```python
from build123d import *

# Parameters (mm, degrees)
SKETCH001_W                   = 50
SKETCH001_H                   = 60
PAD001_DEPTH                  = 17.5
THICKNESS_T                   = -2.5
SKETCH002_R                   = 2.5
PAD002_DEPTH                  = 17.45
SKETCH003_R                   = 0.4
POCKET_DEPTH                  = 1
SKETCH004_W                   = 7
SKETCH004_H                   = 7
PAD003_DEPTH                  = 15
SKETCH004_MIRRORED_2_W        = 7
SKETCH004_MIRRORED_2_H        = 7
PAD003_MIRRORED_2_DEPTH       = 15
SKETCH005_R                   = 1.25
POCKET001_DEPTH               = 12.5
SKETCH005_MIRRORED002_2_R     = 1.25
POCKET001_MIRRORED002_2_DEPTH = 12.5
POCKET002_DEPTH               = 2.5
SKETCH007_W                   = 9
SKETCH007_H                   = 7
POCKET003_DEPTH               = 2.5
FILLET_R                      = 3
FILLET001_R                   = 2
FILLET002_R                   = 1
FILLET003_R                   = 1
FILLET004_R                   = 1
FILLET005_R                   = 1


with BuildPart() as part:
    # Sketch001 → Pad001 (new body)
    with BuildSketch(Plane.XY):
        Rectangle(SKETCH001_W, SKETCH001_H)
    extrude(amount=PAD001_DEPTH)

    # Thickness
    thickness_openings = [part.faces().sort_by_distance(p)[0] for p in [
        (0, 0, 17.5),
    ]]
    offset(amount=THICKNESS_T, openings=thickness_openings)

    # Sketch002 (on Face11 of Thickness) → Pad002 (join)
    with BuildSketch(Plane.XY.offset(2.5)):
        with Locations((-10.415, -7.665)):
            Circle(SKETCH002_R)
        with Locations((-1.695, 13.555)):
            Circle(SKETCH002_R)
    extrude(amount=PAD002_DEPTH)

    # Sketch003 (on Face14 of Pad002) → Pocket (cut)
    with BuildSketch(Plane.XY.offset(19.95)):
        with Locations((-10.415, -7.665)):
            Circle(SKETCH003_R)
        with Locations((-1.695, 13.555)):
            Circle(SKETCH003_R)
    extrude(amount=-POCKET_DEPTH, mode=Mode.SUBTRACT)

    # Sketch004 (on Face11 of Pocket) → Pad003 (join)
    with BuildSketch(Plane.XY.offset(2.5)):
        with Locations((-19, 24)):
            Rectangle(SKETCH004_W, SKETCH004_H)
    pad003 = extrude(amount=PAD003_DEPTH)

    # Sketch004 Mirrored 2 → Pad003 Mirrored 2 (add)
    with BuildSketch(Plane(origin=(0, 0, 2.5), x_dir=(-1, 0, 0), z_dir=(0, 0, -1))):
        with Locations((-19, 24)):
            Rectangle(SKETCH004_MIRRORED_2_W, SKETCH004_MIRRORED_2_H)
    pad003_mirrored_2 = extrude(amount=-PAD003_MIRRORED_2_DEPTH)

    # Mirrored001: Pad003, Pad003 Mirrored 2 across Sketch004 H_Axis
    add(pad003.mirror(Plane(origin=(0, 0, 2.5), x_dir=(0, 0, 1), z_dir=(0, 1, 0))))
    add(pad003_mirrored_2.mirror(Plane(origin=(0, 0, 2.5), x_dir=(0, 0, 1), z_dir=(0, 1, 0))))

    # Sketch005 (on Face11 of MultiTransform) → Pocket001 (cut)
    with BuildSketch(Plane.XY.offset(17.5)):
        with Locations((-19, 24)):
            Circle(SKETCH005_R)
    pocket001 = extrude(amount=-POCKET001_DEPTH, mode=Mode.SUBTRACT)

    # Sketch005 Mirrored002 2 → Pocket001 Mirrored002 2 (cut)
    with BuildSketch(Plane(origin=(0, 0, 17.5), x_dir=(-1, 0, 0), z_dir=(0, 0, -1))):
        with Locations((-19, 24)):
            Circle(SKETCH005_MIRRORED002_2_R)
    pocket001_mirrored002_2 = extrude(amount=POCKET001_MIRRORED002_2_DEPTH, mode=Mode.SUBTRACT)

    # Mirrored003: Pocket001, Pocket001 Mirrored002 2 across Sketch005 H_Axis
    add(pocket001.mirror(Plane(origin=(0, 0, 17.5), x_dir=(0, 0, 1), z_dir=(0, 1, 0))), mode=Mode.SUBTRACT)
    add(pocket001_mirrored002_2.mirror(Plane(origin=(0, 0, 17.5), x_dir=(0, 0, 1), z_dir=(0, 1, 0))), mode=Mode.SUBTRACT)

    # Sketch006 (on Face6 of MultiTransform001) → Pocket002 (cut)
    with BuildSketch(Plane.XZ.offset(30)):
        with BuildLine():
            ThreePointArc((15, 17.5), (10, 22.5), (5, 17.5))
            Line((5, 17.5), (5, 12.5))
            ThreePointArc((5, 12.5), (10, 7.5), (15, 12.5))
            Line((15, 12.5), (15, 17.5))
        make_face()
    extrude(amount=-POCKET002_DEPTH, mode=Mode.SUBTRACT)

    # Sketch007 (on Face1 of Pocket002) → Pocket003 (cut)
    with BuildSketch(Plane(origin=(0, 30, 0), x_dir=(-1, 0, 0), z_dir=(0, 1, 0))):
        with Locations((11, 14)):
            Rectangle(SKETCH007_W, SKETCH007_H)
    extrude(amount=-POCKET003_DEPTH, mode=Mode.SUBTRACT)

    # Fillet
    fillet_edges = [part.edges().sort_by_distance(p)[0] for p in [
        (-12.915, -7.665, 2.5),
        (-4.195, 13.555, 2.5),
    ]]
    fillet(fillet_edges, radius=FILLET_R)

    # Fillet001
    fillet001_edges = [part.edges().sort_by_distance(p)[0] for p in [
        (-25, 0, 0),
        (0, -30, 0),
        (25, 0, 0),
        (0, 30, 0),
    ]]
    fillet(fillet001_edges, radius=FILLET001_R)

    # Fillet002
    fillet002_edges = [part.edges().sort_by_distance(p)[0] for p in [
        (-25, -30, 9.75),
        (25, -30, 9.75),
        (25, 30, 9.75),
        (-25, 30, 9.75),
    ]]
    fillet(fillet002_edges, radius=FILLET002_R)

    # Fillet003
    fillet003_edges = [part.edges().sort_by_distance(p)[0] for p in [
        (-11, 30, 10.5),
        (-15.5, 30, 14),
        (-6.5, 30, 14),
        (-6.5, 27.5, 14),
        (-11, 27.5, 10.5),
    ]]
    fillet(fillet003_edges, radius=FILLET003_R)

    # Fillet004
    fillet004_edges = [part.edges().sort_by_distance(p)[0] for p in [
        (10, -30, 7.5),
        (5, -30, 15),
        (15, -30, 15),
    ]]
    fillet(fillet004_edges, radius=FILLET004_R)

    # Fillet005
    fillet005_edges = [part.edges().sort_by_distance(p)[0] for p in [
        (19, -20.5, 2.5),
        (15.5, -24, 2.5),
        (-15.5, -24, 2.5),
        (-19, -20.5, 2.5),
        (-15.5, 24, 2.5),
        (-19, 20.5, 2.5),
        (19, 20.5, 2.5),
        (15.5, 24, 2.5),
        (0, 27.5, 2.5),
        (22.5, 0, 2.5),
        (0, -27.5, 2.5),
        (-22.5, 0, 2.5),
    ]]
    fillet(fillet005_edges, radius=FILLET005_R)


solid = part.part
```
Geometry: final body of the model. Coordinates: model frame, mm. A direction names the side the tool comes from. Coordinates: 2 decimals unless noted, no trailing zeros. Order: outer loops, then holes, each group sorted by start corner. A loop starts at its lowest first (then second) coordinate and runs counter-clockwise, first axis right, second up. Notation, with made-up numbers: (47.25, 41.25) -> (64.25, 41.25) arc R23 cw to (64.25, 57.25) -> close; hole circle Ø2 at (-10.5, 25). An arc over 180 degrees is marked (long way). Write item = value, one per line.
(1) Cut plane A-A on y = 6. Return loops of the section in (x, z).
Solved:
outline = (-25, 2) arc R2 ccw to (-23, 0) -> (23, 0) arc R2 ccw to (25, 2) -> (25, 17.5) -> (22.5, 17.5) -> (22.5, 3.5) arc R1 cw to (21.5, 2.5) -> (-21.5, 2.5) arc R1 cw to (-22.5, 3.5) -> (-22.5, 17.5) -> (-25, 17.5) -> close
(2) Line query: line 1 (Y direction, x = -19, z = 10.75); line 2 (X direction, y = -24, z = 13.5); line 3 (X direction, y = -11, z = 6.5). Output: solid intervals per line, ascending.
Solved:
line_1 = -30 to -25.25, -22.75 to -20.5, 20.5 to 22.75, 25.25 to 30
line_2 = -25 to -20.25, -17.75 to -15.5, 15.5 to 17.75, 20.25 to 25
line_3 = -25 to -22.5, 22.5 to 25
(3) Cut plane D-D on y = -24. Return loops of the section in (x, z), plus the area to 3 significant figures.
Solved:
outline = (-25, 2) arc R2 ccw to (-23, 0) -> (23, 0) arc R2 ccw to (25, 2) -> (25, 17.5) -> (20.25, 17.5) -> (20.25, 5) -> (17.75, 5) -> (17.75, 17.5) -> (15.5, 17.5) -> (15.5, 3.5) arc R1 cw to (14.5, 2.5) -> (-14.5, 2.5) arc R1 cw to (-15.5, 3.5) -> (-15.5, 17.5) -> (-17.75, 17.5) -> (-17.75, 5) -> (-20.25, 5) -> (-20.25, 17.5) -> (-25, 17.5) -> close
area = 346 mm²
(4) Cut plane B-B on x = 10. Return loops of the section in (y, z), plus the area to 3 significant figures.
Solved:
outline = (-30, 2) arc R2 ccw to (-28, 0) -> (28, 0) arc R2 ccw to (30, 2) -> (30, 17.5) -> (27.5, 17.5) -> (27.5, 3.5) arc R1 cw to (26.5, 2.5) -> (-26.5, 2.5) arc R1 cw to (-27.5, 3.5) -> (-27.5, 7.5) -> (-29, 7.5) arc R1 ccw to (-30, 6.5) -> close
area = 198 mm²
(5) Pin query (flat end, axial travel): pin 1 Ø2 at (x, y) = (19, -24.5) entering from +Z; pin 2 Ø3 at (x, y) = (-12, 14) entering from +Z. Return the tip coordinate at first contact, or that it passes through.
Solved:
pin_1 = 17.5
pin_2 = 2.5
(6) Cut plane C-C on z = 15.25. Count the separate pieces of the cut face and the enclosed holes in it, plus the area to 3 significant figures.
Solved:
separate_pieces = 4
enclosed_holes = 4
area = 691 mm²
(7) Access query for faces 1 (the flat face through (3, 27.5, 10)), 2 (the cylindrical face through (-24.43, 0.41, 0.6)), 3 (the flat face through (5, -28, 15)). Directions: +Z, -Z, +X, -X, +Y, -Y. A direction counts if a zero-diameter tool reaches every point of the face in a straight line with its end or side. Return the directions, or none.
Solved:
face_1 = +Z
face_2 = -Z, -X, +Y, -Y
face_3 = +Z, -Y
